```python
from build123d import *

# Parameters (mm, degrees)
BOSS_EXTRU_1_DEPTH           = 137
ESQUISSE2_R                  = 32
BOSS_EXTRU_2_DEPTH           = 7
ESQUISSE3_R                  = 27
BOSS_EXTRU_3_DEPTH           = 13
ESQUISSE4_R                  = 7
BOSS_EXTRU_4_DEPTH           = 32
ENL_V_MAT_EXTRU_1_DEPTH      = 206.475667659
ENL_V_MAT_EXTRU_1_DEPTH_BACK = 206.475667659
ESQUISSE5_R                  = 3.25


with BuildPart() as part:
    # Esquisse1 → Boss.-Extru.1 (new body)
    with BuildSketch(Plane.XY):
        Polygon((-47, 0), (47, 0), (47, 11.5), (35, 11.5), (35, 77), (-35, 77), (-35, 11.5), (-47, 11.5), align=None)
    extrude(amount=BOSS_EXTRU_1_DEPTH)

    # Esquisse2 → Boss.-Extru.2 (add)
    with BuildSketch(Plane.XY.offset(137)):
        with Locations((0, 38.5)):
            Circle(ESQUISSE2_R)
    extrude(amount=BOSS_EXTRU_2_DEPTH)

    # Esquisse3 → Boss.-Extru.3 (add)
    with BuildSketch(Plane.XY.offset(144)):
        with Locations(Location((0, 38.5, 0), (0, 0, 180))):
            Circle(ESQUISSE3_R)
    extrude(amount=BOSS_EXTRU_3_DEPTH)

    # Esquisse4 → Boss.-Extru.4 (add)
    with BuildSketch(Plane.XY.offset(157)):
        with Locations((0, 38.5)):
            Circle(ESQUISSE4_R)
    extrude(amount=BOSS_EXTRU_4_DEPTH)

    # Esquisse5 → Enlèv. mat.-Extru.1 (cut, two sides: drawn at the far end of the back side and taken through both)
    with BuildSketch(Plane(origin=(0, 11.5, 0), x_dir=(1, 0, 0), z_dir=(0, 1, 0)).offset(-ENL_V_MAT_EXTRU_1_DEPTH_BACK)):
        with Locations(Location((40.5, -122, 0), (0, 0, 270))):
            Circle(ESQUISSE5_R)
        with Locations(Location((40.5, -87, 0), (0, 0, 270))):
            Circle(ESQUISSE5_R)
        with Locations(Location((40.5, -52, 0), (0, 0, 270))):
            Circle(ESQUISSE5_R)
        with Locations(Location((40.5, -17, 0), (0, 0, 270))):
            Circle(ESQUISSE5_R)
        with Locations(Location((-40.5, -17, 0), (0, 0, 90))):
            Circle(ESQUISSE5_R)
        with Locations(Location((-40.5, -52, 0), (0, 0, 90))):
            Circle(ESQUISSE5_R)
        with Locations(Location((-40.5, -87, 0), (0, 0, 90))):
            Circle(ESQUISSE5_R)
        with Locations(Location((-40.5, -122, 0), (0, 0, 90))):
            Circle(ESQUISSE5_R)
    extrude(amount=ENL_V_MAT_EXTRU_1_DEPTH + ENL_V_MAT_EXTRU_1_DEPTH_BACK, mode=Mode.SUBTRACT)


solid = part.part
```
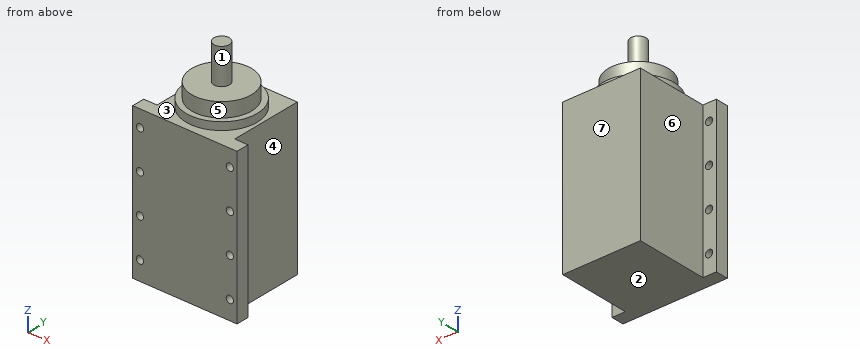
Verification items for the finished model (mm, model axes). Face numbers are marked on the shaded views. A direction names the side the tool comes from. Coordinates: 2 decimals unless noted, no trailing zeros. Loops run counter-clockwise (first coordinate to the right, second up) from the corner with the lowest first, then second, coordinate; pieces in that order, holes last. Notation, with made-up numbers: (-14.5, 13.5) - (-4.5, 13.5) arc R24 ccw to (-4.5, 42.5) - close; hole circle Ø10 at (59.5, 69.5). An arc over 180 degrees is marked (long way). Put each result on its own line as item: value.
Item 1: Section check A-A (x = 40.5). Enter the section's corners in (y, z).
Conclusion:
outline: (0, 0) - (11.5, 0) - (11.5, 13.75) - (0, 13.75) - close; (0, 20.25) - (11.5, 20.25) - (11.5, 48.75) - (0, 48.75) - close; (0, 55.25) - (11.5, 55.25) - (11.5, 83.75) - (0, 83.75) - close; (0, 90.25) - (11.5, 90.25) - (11.5, 118.75) - (0, 118.75) - close; (0, 125.25) - (11.5, 125.25) - (11.5, 137) - (0, 137) - close
Item 2: Gauge pin test, flat ends, axial feed: pin 1 Ø5 at (y, z) = (21, 33) entering from +X; pin 2 Ø23 at (x, y) = (20, 30.5) entering from +Z; pin 3 Ø8 at (y, z) = (46, 142) entering from -X. Record the tip position at first contact, or that the pin passes through.
Conclusion:
pin 1: stops at x = 35
pin 2: stops at z = 157
pin 3: stops at x = -31.81
Item 3: Scan lines: line 1 along X through (y, z) = (7.75, 122); line 2 along Z through (x, y) = (40, 3); line 3 along Z through (x, y) = (-14, 14). Record each from-to range of solid material in increasing order.
Conclusion:
line 1: x = -47 to -43.75, -37.25 to 37.25, 43.75 to 47
line 2: z = 0 to 13.79, 20.21 to 48.79, 55.21 to 83.79, 90.21 to 118.79, 125.21 to 137
line 3: z = 0 to 144
Item 4: Draft check along Z on the marked faces 1, 2 and 3. Enter one of: pulls with the +Z half, pulls with the -Z half, needs draft (parallel to the pull), parting line crosses it, or undercut.
Conclusion:
face 1: needs draft
face 2: pulls with the -Z half
face 3: pulls with the +Z half
Item 5: Set-up check for the marked faces 4, 5, 6 and 7: record each of +Z, -Z, +X, -X, +Y, -Y from which the full face is reachable in a straight line by a thin tool's end or side.
Conclusion:
face 4: +Z, -Z, +X, +Y
face 5: +Z
face 6: +Z, -Z, -X, +Y
face 7: +Z, -Z, +X, -X, +Y
Item 6: Section check B-B (z = 87). Enter the section's corners in (x, y), then the cut area to 3 significant figures.
Conclusion:
outline: (-47, 0) - (-43.75, 0) - (-43.75, 11.5) - (-47, 11.5) - close; (-37.25, 0) - (37.25, 0) - (37.25, 11.5) - (35, 11.5) - (35, 77) - (-35, 77) - (-35, 11.5) - (-37.25, 11.5) - close; (43.75, 0) - (47, 0) - (47, 11.5) - (43.75, 11.5) - close
area: 5,520 mm2
Item 7: Section check D-D (x = 0). Enter the section's corners in (y, z), then the cut area to 3 significant figures.
Conclusion:
outline: (0, 0) - (77, 0) - (77, 137) - (70.5, 137) - (70.5, 144) - (65.5, 144) - (65.5, 157) - (45.5, 157) - (45.5, 189) - (31.5, 189) - (31.5, 157) - (11.5, 157) - (11.5, 144) - (6.5, 144) - (6.5, 137) - (0, 137) - close
area: 12,100 mm2
Item 8: Section check C-C (y = 38.5). Enter the section's corners in (x, z).
Conclusion:
outline: (-35, 0) - (35, 0) - (35, 137) - (32, 137) - (32, 144) - (27, 144) - (27, 157) - (7, 157) - (7, 189) - (-7, 189) - (-7, 157) - (-27, 157) - (-27, 144) - (-32, 144) - (-32, 137) - (-35, 137) - close
